from build123d import *

# Parameters (mm, degrees)
F1_DEPTH  = 57.15
F3_DEPTH  = 7.874
F5_DEPTH  = 7.874
F6_R      = 9.92251
F7_DEPTH  = 25.4
F8_R      = 9.92251
F9_DEPTH  = 25.4
F10_W     = 76.2
F10_H     = 44.45
F11_DEPTH = 7.9375
F12_R     = 10.3251
F13_DEPTH = 25.4
F14_R     = 6.35


with BuildPart() as f1:
    # F0 (on Right) → F1 (new body)
    with BuildSketch(Plane.YZ):
        with BuildLine():
            ThreePointArc((-12.7, 12.7), (-8.9802561211, 3.7197438789), (0, 0))
            Line((0, 0), (63.5, 0))
            ThreePointArc((63.5, 0), (72.4802561211, 3.7197438789), (76.2, 12.7))
            Line((76.2, 12.7), (76.2, 57.15))
            Line((76.2, 57.15), (68.2625, 57.15))
            Line((68.2625, 57.15), (68.2625, 12.7))
            ThreePointArc((68.2625, 12.7), (66.8675960454, 9.3324039546), (63.5, 7.9375))
            Line((63.5, 7.9375), (0, 7.9375))
            ThreePointArc((0, 7.9375), (-3.3675960454, 9.3324039546), (-4.7625, 12.7))
            Line((-4.7625, 12.7), (-4.7625, 57.15))
            Line((-4.7625, 57.15), (-12.7, 57.15))
            Line((-12.7, 57.15), (-12.7, 12.7))
        make_face()
    extrude(amount=F1_DEPTH)

    # F2 (on face) → F3 (join)
    with BuildSketch(Plane.XZ.offset(12.7)):
        with BuildLine():
            Line((0, 57.15), (57.15, 57.15))
            ThreePointArc((57.15, 57.15), (28.575, 85.725), (0, 57.15))
        make_face()
    extrude(amount=-F3_DEPTH)

    # F4 (on face) → F5 (join)
    with BuildSketch(Plane(origin=(0, 76.2, 0), x_dir=(-1, 0, 0), z_dir=(0, 1, 0))):
        with BuildLine():
            Line((-57.15, 57.15), (0, 57.15))
            ThreePointArc((0, 57.15), (-28.575, 85.725), (-57.15, 57.15))
        make_face()
    extrude(amount=-F5_DEPTH)

    # F6 (on face) → F7 (cut)
    with BuildSketch(Plane.XZ.offset(12.7)):
        with Locations((28.575, 57.15)):
            Circle(F6_R)
    extrude(amount=-F7_DEPTH, mode=Mode.SUBTRACT)

    # F8 (on face) → F9 (cut)
    with BuildSketch(Plane(origin=(0, 76.2, 0), x_dir=(-1, 0, 0), z_dir=(0, 1, 0))):
        with Locations((-28.575, 57.15)):
            Circle(F8_R)
    extrude(amount=-F9_DEPTH, mode=Mode.SUBTRACT)

    # F10 (on face) → F11 (join)
    with BuildSketch(Plane.XY.offset(7.9375)):
        with Locations((95.25, 31.75)):
            Rectangle(F10_W, F10_H)
    extrude(amount=-F11_DEPTH)

    # F12 (on face) → F13 (cut)
    with BuildSketch(Plane.XY.offset(7.9375)):
        with Locations((73.025, 31.75)):
            Circle(F12_R)
        with Locations((111.125, 31.75)):
            Circle(F12_R)
        with BuildLine():
            ThreePointArc((111.125, 53.975), (126.8404482119, 47.4654482119), (133.35, 31.75))
            Line((133.35, 31.75), (133.35, 53.975))
            Line((133.35, 53.975), (111.125, 53.975))
        make_face()
        with BuildLine():
            Line((133.35, 9.525), (133.35, 31.75))
            ThreePointArc((133.35, 31.75), (126.8404482119, 16.0345517881), (111.125, 9.525))
            Line((111.125, 9.525), (133.35, 9.525))
        make_face()
    extrude(amount=-F13_DEPTH, mode=Mode.SUBTRACT)

    # F14
    f14_edges = [f1.edges().sort_by_distance(p)[0] for p in [
        (57.15, 9.525, 3.96875),
        (57.15, 53.975, 3.96875),
    ]]
    fillet(f14_edges, radius=F14_R)


solid = f1.part
Build history of the part. All positions in model axes, mm. A direction names the side the tool comes from. Coordinates: 2 decimals unless noted, no trailing zeros. Order: outer loops, then holes, each group sorted by start corner. A loop starts at its lowest first (then second) coordinate and runs counter-clockwise, first axis right, second up. Notation, with made-up numbers: (13.5, -19.5) -> (20.5, -19.5) arc R25 cw to (20.5, 13.5) -> close; hole circle Ø1 at (61.25, -3). An arc over 180 degrees is marked (long way). One line per item, written item: value.
(1) Slice it at B-B, the plane y = 38. List the corners of the cut face in (x, z).
Checked values:
outline: (0, 0) -> (64.81, 0) -> (64.81, 7.94) -> (0, 7.94) -> close; (81.24, 0) -> (102.91, 0) -> (102.91, 7.94) -> (81.24, 7.94) -> close; (119.34, 0) -> (132.45, 0) -> (132.45, 7.94) -> (119.34, 7.94) -> close
(2) Slice it at C-C, the plane x = 80.5. List the corners of the cut face in (y, z) (1 decimal), plus the area to 3 significant figures.
Checked values:
outline: (9.5, 0) -> (24.6, 0) -> (24.6, 7.9) -> (9.5, 7.9) -> close; (38.9, 0) -> (54, 0) -> (54, 7.9) -> (38.9, 7.9) -> close
area: 240 mm2
(3) Drop flat-ended pins along their axis: pin 1 Ø12.5 at (y, z) = (-6.5, 26.5) entering from +X; pin 2 Ø23.5 at (x, y) = (111.125, 31.75) entering from +Z. Give the stop position or say it passes through.
Checked values:
pin 1: x = 57.15
pin 2: z = 7.94
(4) Tool access for faces 5 (the cylindrical face through (28.17, 72.38, 3.62)), 6 (the flat face through (87, 9.525, 4)), 7 (the flat face through (28, -4.762, 35)), 8 (the flat face through (57.15, 72, 29)): list every direction of +Z, -Z, +X, -X, +Y, -Y with a clear straight run to the whole face (end or side of a thin tool).
Checked values:
face 5: -Z, +X, -X, +Y
face 6: +Z, -Z, +X, -Y
face 7: +Z, +X, -X
face 8: +Z, -Z, +X, +Y
(5) Mould opens along Y. For faces 1 (the cylindrical face through (26.424, -8.787, 47.463)), 2 (the cylindrical face through (62.71, 32.2, 4.02)), 3 (the flat face through (87, 53.975, 4)), 4 (the flat face through (28, -12.7, 42)) say: pulls with the +Y half, pulls with the -Y half, needs draft (parallel to the pull), parting line crosses it, or undercut.
Checked values:
face 1: needs draft
face 2: undercut
face 3: pulls with the +Y half
face 4: pulls with the -Y half
(6) Slice it at D-D, the plane z = 62. List the corners of the cut face in (x, y), plus the area to 3 significant figures.
Checked values:
outline: (0.41, -12.7) -> (19.92, -12.7) -> (19.92, -4.83) -> (0.41, -4.83) -> close; (0.41, 68.33) -> (19.92, 68.33) -> (19.92, 76.2) -> (0.41, 76.2) -> close; (37.23, -12.7) -> (56.74, -12.7) -> (56.74, -4.83) -> (37.23, -4.83) -> close; (37.23, 68.33) -> (56.74, 68.33) -> (56.74, 76.2) -> (37.23, 76.2) -> close
area: 614 mm2
(7) Slice it at A-A, the plane z = 40. List the corners of the cut face in (x, y).
Checked values:
outline: (0, -12.7) -> (57.15, -12.7) -> (57.15, -4.76) -> (0, -4.76) -> close; (0, 68.26) -> (57.15, 68.26) -> (57.15, 76.2) -> (0, 76.2) -> close
(8) Probe line 1 (X direction, y = 74.5, z = 57.15); line 2 (X direction, y = 31, z = 2); line 3 (Y direction, x = 56, z = 28). List the from-to ranges inside material, lowest first. Write a range as [from, to].
Checked values:
line 1: [0, 18.65], [38.5, 57.15]
line 2: [0, 62.73], [83.32, 100.83], [121.42, 133.34]
line 3: [-12.7, -4.76], [68.26, 76.2]
